Part model, mm, in its own coordinate system. A direction names the side the tool comes from. Round coordinates to 2 decimals unless told otherwise and drop trailing zeros. Order: outer loops, then holes, each group sorted by start corner. A loop starts at its lowest first (then second) coordinate and runs counter-clockwise, first axis right, second up. Notation, with made-up numbers: (-12, 64.5) - (12, 64.5) arc R29 cw to (12, 86.5) - close; hole circle Ø5 at (66, 21). An arc over 180 degrees is marked (long way). Return JSON: item names as keys, results as strings. Group by question number.
Item 1: Saw through at C-C on y = 12.5. List the corners of the cut face in (x, z) (3 decimals).
Item 2: Saw through at A-A on y = 17. List the corners of the cut face in (x, z), and give its area (3 significant figures).
Item 3: Drop flat-ended pins along their axis: pin 1 (12 mm diameter, centred on x = -1.5, z = -6, fed in from -Y); pin 2 (0.6 mm diameter, centred on y = 16, z = 2, fed in from -X); pin 3 (3 mm diameter, centred on y = 10.5, z = -6.5, fed in from +X); pin 4 (0.8 mm diameter, centred on x = -17.5, y = 16.5, fed in from -Z). Give the stop position or say it passes through.
Item 4: Saw through at B-B on x = 8.6. List the corners of the cut face in (y, z).
Item 5: Tool access for faces 1 (the face through (13.6, 16.5, 1.9)), 2 (the face through (13.7, 16.5, -1.9)), 3 (the face through (-1, 2, 0)): list every direction of +Z, -Z, +X, -X, +Y, -Y with a clear straight run to the whole face (end or side of a thin tool).
Item 6: Probe probe 1 along Z at (x, y) = (8.6, 1.55); probe 2 along X at (y, z) = (1.4, 5.55); probe 3 along Y at (x, z) = (-13, 2.5). List the from-to ranges inside material, lowest first.
Item 7: Saw through at D-D on z = -0.5. List the corners of the cut face in (x, y), and give its area (3 significant figures).
Item 8: Two-plate mould, pull along X, no slides. Class faces 4 (the face through (11.75, 14, 0)), 5 (the face through (13, 7, -7.7)): released by +X, released by -X, zero draft, split by the parting line, or undercut.
```python
from build123d import *
from build123d.topology import SkipClean

# Parameters (mm, degrees)
SALIENTE_EXTRUIR1_DEPTH           = 14.8
CORTAR_EXTRUIR1_DEPTH             = 25.86366797
CORTAR_EXTRUIR1_DEPTH_BACK        = 25.86366797
CROQUIS2_W                        = 15.4
CROQUIS2_H                        = 11
CORTAR_EXTRUIR2_REACH             = 26.864
CORTAR_EXTRUIR2_DIRECTION_2_DEPTH = 25.86366797
SALIENTE_EXTRUIR2_DEPTH           = 3.5
CROQUIS5_R                        = 1.1
CORTAR_EXTRUIR3_DEPTH             = 26.784723868
CORTAR_EXTRUIR4_DEPTH             = 26.784723868
CROQUIS7_W                        = 27.231493877
CROQUIS7_H                        = 23.409529823
CORTAR_EXTRUIR5_DEPTH             = 28.093393751
CROQUIS8_W                        = 20.5
CROQUIS8_H                        = 2
SALIENTE_EXTRUIR3_DEPTH           = 0.5


with BuildPart() as part:
    # Croquis1 → Saliente-Extruir1 (new body)
    with BuildSketch(Plane(origin=(0, 0, 0), x_dir=(1, 0, 0), z_dir=(0, 1, 0))):
        with BuildLine():
            Line((-13.935, -10.25), (13.935, -10.25))
            ThreePointArc((13.935, -10.25), (17.149328994, 0), (13.935, 10.25))
            Line((13.935, 10.25), (-13.935, 10.25))
            ThreePointArc((-13.935, 10.25), (-17.149328994, 0), (-13.935, -10.25))
        make_face()
    extrude(amount=SALIENTE_EXTRUIR1_DEPTH)

    # Croquis2 → Cortar-Extruir1 (cut, two sides: drawn at the far end of the back side and taken through both)
    with BuildSketch(Plane(origin=(0, 0, 0), x_dir=(0, 0, -1), z_dir=(1, 0, 0)).offset(-CORTAR_EXTRUIR1_DEPTH_BACK)):
        with Locations((0, 7.5)):
            Rectangle(CROQUIS2_W, CROQUIS2_H)
    extrude(amount=CORTAR_EXTRUIR1_DEPTH + CORTAR_EXTRUIR1_DEPTH_BACK, mode=Mode.SUBTRACT)

    # Cortar-Extruir2: up to this face of the body (flat: up to its plane)
    cortar_extruir2_end = Plane(part.part.faces().sort_by_distance((0, 2, 0))[0])
    # Croquis3 → Cortar-Extruir2 (cut, up to the picked face)
    with BuildSketch(Plane(origin=(0, 14.8, 0), x_dir=(1, 0, 0), z_dir=(0, 1, 0)), mode=Mode.PRIVATE) as cortar_extruir2_sk1:
        Polygon((10.9, -10.25), (-10.9, -10.25), (-10.9, -4.5), (-11.75, -4.5), (-11.75, 4.5), (-10.9, 4.5), (-10.9, 10.25), (10.9, 10.25), (10.9, 4.5), (11.75, 4.5), (11.75, -4.5), (10.9, -4.5), align=None)
    cortar_extruir2_tool1 = split(extrude(cortar_extruir2_sk1.sketch, amount=-CORTAR_EXTRUIR2_REACH, mode=Mode.PRIVATE), bisect_by=cortar_extruir2_end, keep=Keep.BOTH, mode=Mode.PRIVATE)
    add(cortar_extruir2_tool1.solids().sort_by(Axis((0, 14.8, 0), (0, -1, 0)))[0], mode=Mode.SUBTRACT)

    # Croquis3 → Cortar-Extruir2 direction 2 (cut)
    with BuildSketch(Plane(origin=(0, 14.8, 0), x_dir=(1, 0, 0), z_dir=(0, 1, 0))):
        Polygon((10.9, -10.25), (-10.9, -10.25), (-10.9, -4.5), (-11.75, -4.5), (-11.75, 4.5), (-10.9, 4.5), (-10.9, 10.25), (10.9, 10.25), (10.9, 4.5), (11.75, 4.5), (11.75, -4.5), (10.9, -4.5), align=None)
    extrude(amount=CORTAR_EXTRUIR2_DIRECTION_2_DEPTH, mode=Mode.SUBTRACT)

    # Croquis4 → Saliente-Extruir2 (add)
    with SkipClean():  # the faces are left unmerged after this step: merging them gives an invalid solid
        with BuildSketch(Plane(origin=(0, 14.8, 0), x_dir=(1, 0, 0), z_dir=(0, 1, 0))):
            with BuildLine():
                Line((-13.2, 1.9), (-13.2, -1.9))
                Line((-13.2, -1.9), (-14.1, -1.9))
                Line((-14.1, -1.9), (-14.1, -2.4))
                Line((-14.1, -2.4), (-15.5, -2.4))
                Line((-15.5, -2.4), (-15.5, -1.9))
                Line((-15.5, -1.9), (-17.048488638, -1.9))
                ThreePointArc((-17.048488638, -1.9), (-17.149328994, 0), (-17.048488638, 1.9))
                Line((-17.048488638, 1.9), (-15.5, 1.9))
                Line((-15.5, 1.9), (-15.5, 2.4))
                Line((-15.5, 2.4), (-14.1, 2.4))
                Line((-14.1, 2.4), (-14.1, 1.9))
                Line((-14.1, 1.9), (-13.2, 1.9))
            make_face()
        saliente_extruir2 = extrude(amount=SALIENTE_EXTRUIR2_DEPTH)

    # Simetría1: Saliente-Extruir2 across plane
    with SkipClean():  # the faces are left unmerged after this step: merging them gives an invalid solid
        add(saliente_extruir2.mirror(Plane(origin=(0, 0, 0), x_dir=(0, 0, 1), z_dir=(1, 0, 0))))

    # Croquis5 → Cortar-Extruir3 (cut, through all)
    with SkipClean():  # the faces are left unmerged after this step: merging them gives an invalid solid
        with BuildSketch(Plane(origin=(0, 2, 0), x_dir=(1, 0, 0), z_dir=(0, 1, 0))):
            with Locations(Location((-8.6, -5.55, 0), (0, 0, 270))):
                Circle(CROQUIS5_R)
            with Locations(Location((-8.6, 5.55, 0), (0, 0, 270))):
                Circle(CROQUIS5_R)
            with Locations(Location((8.6, -5.55, 0), (0, 0, 90))):
                Circle(CROQUIS5_R)
            with Locations(Location((8.6, 5.55, 0), (0, 0, 90))):
                Circle(CROQUIS5_R)
        extrude(amount=-CORTAR_EXTRUIR3_DEPTH, mode=Mode.SUBTRACT)

    # Croquis6 → Cortar-Extruir4 (cut, through all)
    with BuildSketch(Plane(origin=(0, 2, 0), x_dir=(1, 0, 0), z_dir=(0, 1, 0))):
        with BuildLine():
            Line((-13.156952885, 7.7), (-13.156952885, -7.7))
            Line((-13.156952885, -7.7), (-15.413905769, -7.7))
            ThreePointArc((-15.413905769, -7.7), (-17.149328994, 0), (-15.413905769, 7.7))
            Line((-15.413905769, 7.7), (-13.156952885, 7.7))
        make_face()
        with BuildLine():
            Line((13.156952885, 7.7), (13.156952885, -7.7))
            Line((13.156952885, -7.7), (15.413905769, -7.7))
            ThreePointArc((15.413905769, -7.7), (17.149328994, 0), (15.413905769, 7.7))
            Line((15.413905769, 7.7), (13.156952885, 7.7))
        make_face()
    extrude(amount=-CORTAR_EXTRUIR4_DEPTH, mode=Mode.SUBTRACT)

    # Croquis7 → Cortar-Extruir5 (cut, through all)
    with BuildSketch(Plane(origin=(0, 0, 0), x_dir=(0, 0, -1), z_dir=(1, 0, 0))):
        with Locations((0.238872753, 8.562005531)):
            Rectangle(CROQUIS7_W, CROQUIS7_H)
    extrude(amount=-CORTAR_EXTRUIR5_DEPTH, mode=Mode.SUBTRACT)

    # Croquis8 → Saliente-Extruir3 (add)
    with BuildSketch(Plane.ZY):
        with Locations((0, 1)):
            Rectangle(CROQUIS8_W, CROQUIS8_H)
    extrude(amount=SALIENTE_EXTRUIR3_DEPTH)

    # Simetría4: part across plane


with BuildPart() as part_1:
    add(part.part)
    add(part.part.mirror(Plane.ZY.offset(0.5)))


solid = part_1.part
```
Filled in:
{
 "1": {"outline": "(-16.414, -7.7) arc R17.95 ccw to (-14.935, -10.25) - (-11.9, -10.25) - (-11.9, -7.7) - close; (-16.414, 7.7) - (-11.9, 7.7) - (-11.9, 10.25) - (-14.935, 10.25) arc R17.95 ccw to start; (10.9, -10.25) - (13.935, -10.25) arc R17.95 ccw to (15.414, -7.7) - (10.9, -7.7) - close; (10.9, 7.7) - (15.414, 7.7) arc R17.95 ccw to (13.935, 10.25) - (10.9, 10.25) - close"},
 "2": {"outline": "(-18.05, -1.9) - (-16.5, -1.9) - (-16.5, -2.4) - (-15.1, -2.4) - (-15.1, -1.9) - (-14.2, -1.9) - (-14.2, 1.9) - (-15.1, 1.9) - (-15.1, 2.4) - (-16.5, 2.4) - (-16.5, 1.9) - (-18.05, 1.9) arc R17.95 ccw to start; (13.2, -1.9) - (14.1, -1.9) - (14.1, -2.4) - (15.5, -2.4) - (15.5, -1.9) - (17.05, -1.9) arc R17.95 ccw to (17.05, 1.9) - (15.5, 1.9) - (15.5, 2.4) - (14.1, 2.4) - (14.1, 1.9) - (13.2, 1.9) - close", "area": "32.6 mm^2"},
 "3": {"pin 1": "stops at y = 0", "pin 2": "stops at x = -18.07", "pin 3": "stops at x = 15.41", "pin 4": "stops at z = -1.9"},
 "4": {"outline": "(0, -10.25) - (2, -10.25) - (2, -6.65) - (0, -6.65) - close; (0, -4.45) - (2, -4.45) - (2, 4.45) - (0, 4.45) - close; (0, 6.65) - (2, 6.65) - (2, 10.25) - (0, 10.25) - close"},
 "5": {"face 1": "+Z, +Y", "face 2": "-Z, +Y", "face 3": "none"},
 "6": {"probe 1": "z = -10.25 to -6.65, -4.45 to 4.45, 6.65 to 10.25", "probe 2": "x = -14.16 to -10.7, -8.5 to 7.5, 9.7 to 13.16", "probe 3": "y = 0 to 2, 13 to 14.8"},
 "7": {"outline": "(-18.14, 13) - (-12.75, 13) - (-12.75, 14.8) - (-14.2, 14.8) - (-14.2, 18.3) - (-18.14, 18.3) - close; (-14.16, 0) - (13.16, 0) - (13.16, 2) - (-14.16, 2) - close; (11.75, 13) - (17.14, 13) - (17.14, 18.3) - (13.2, 18.3) - (13.2, 14.8) - (11.75, 14.8) - close", "area": "102 mm^2"},
 "8": {"face 4": "undercut", "face 5": "zero draft"}
}
